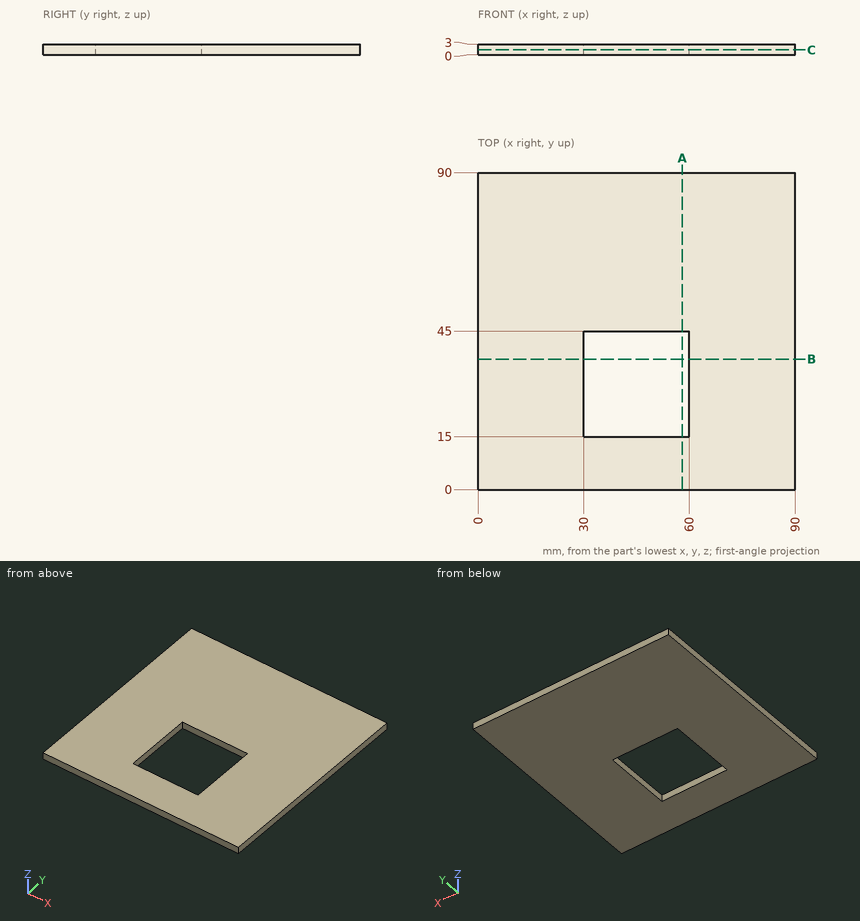
For this review, use the dimensioned drawing (mm, ordinates from the lowest corner) and the shaded views. Give positions to 0.01 mm unless a question says otherwise; leave off trailing zeros. Order: outer loops, then holes, each group sorted by start corner. A loop starts at its lowest first (then second) coordinate and runs counter-clockwise, first axis right, second up. Notation, with made-up numbers: (9, 24.25) - (27, 24.25) arc R14 cw to (27, 33.25) - close; hole circle Ø9 at (9.25, 89). An arc over 180 degrees is marked (long way). Use CSV: the item, a comma, the result in double quotes. Start each with the question number.
Q1. For line 1 (X direction, y = 17.5, z = 1.55); line 2 (Y direction, x = 36.5, z = 2.1), list the stretches that pass through material, from the lowest coordinate up.
Q2. Take a section at B-B (y = 37). State the section outline as (x, z) points.
Q3. Take a section at C-C (z = 1.3). State the section outline as (x, y) points.
Q4. Take a section at A-A (x = 58). State the section outline as (y, z) points.
Q5. For P1, Ø5, axis at x = 17.5, y = 50.5, coming from the -Z side, flat-tipped, find the tip position at first contact; note if it passes through.
Calculated:
1,line 1,"x = 0 to 30, 60 to 90"
1,line 2,"y = 0 to 15, 45 to 90"
2,outline,"(0, 0) - (30, 0) - (30, 3) - (0, 3) - close; (60, 0) - (90, 0) - (90, 3) - (60, 3) - close"
3,outline,"(0, 0) - (90, 0) - (90, 90) - (0, 90) - close; hole (30, 15) - (60, 15) - (60, 45) - (30, 45) - close"
4,outline,"(0, 0) - (15, 0) - (15, 3) - (0, 3) - close; (45, 0) - (90, 0) - (90, 3) - (45, 3) - close"
5,P1,"stops at z = 0"
